```python
from build123d import *

# Parameters (mm, degrees)
BOSS_EXTRUDE2_DEPTH = 11.684
SKETCH3_R           = 12
CUT_EXTRUDE1_DEPTH  = 17.78
SKETCH5_R           = 4.7625
SKETCH5_R_2         = 3.96875
CUT_EXTRUDE3_DEPTH  = 24.368
SKETCH4_R           = 7.5
CUT_EXTRUDE2_DEPTH  = 24.368
CUT_EXTRUDE4_DEPTH  = 9.525
CUT_EXTRUDE5_DEPTH  = 9.525
SKETCH10_R          = 14
CUT_EXTRUDE6_DEPTH  = 1.905
CUT_EXTRUDE7_REACH  = 35.001
SKETCH12_W          = 38.1
SKETCH12_H          = 16.002
CUT_EXTRUDE8_REACH  = 32.013
SKETCH15_W          = 50.8
SKETCH15_H          = 17.5768
FILLET2_R           = 3.175
FILLET3_R           = 6.35
FILLET4_R           = 2.54
SKETCH16_R          = 17.272
CUT_EXTRUDE9_DEPTH  = 3.048


with BuildPart() as part:
    # Sketch2 → Boss-Extrude2 (new body, symmetric)
    with BuildSketch(Plane(origin=(0, 0, 0), x_dir=(1, 0, 0), z_dir=(0, 1, 0))):
        with BuildLine():
            Line((-42.844042296, 9.135566968), (24.187242381, 62.581479461))
            ThreePointArc((24.187242381, 62.581479461), (37.709893542, 62.836755255), (41.463262143, 49.842930403))
            Line((41.463262143, 49.842930403), (19.040802343, -7.451688072))
            ThreePointArc((19.040802343, -7.451688072), (9.340036317, -18.189104722), (-5.038725, -19.816434073))
            Line((-5.038725, -19.816434073), (-38.439271429, -11.323676613))
            ThreePointArc((-38.439271429, -11.323676613), (-46.982276413, -2.459157895), (-42.844042296, 9.135566968))
        make_face()
    extrude(amount=BOSS_EXTRUDE2_DEPTH, both=True)

    # Sketch3 → Cut-Extrude1 (cut)
    with BuildSketch(Plane.XZ.offset(11.684)):
        Circle(SKETCH3_R)
    extrude(amount=-CUT_EXTRUDE1_DEPTH, mode=Mode.SUBTRACT)

    # Sketch5 → Cut-Extrude3 (cut, through all)
    with BuildSketch(Plane(origin=(0, 11.684, 0), x_dir=(1, 0, 0), z_dir=(0, 1, 0))):
        with Locations((-35.56, 0)):
            Circle(SKETCH5_R)
        with Locations((31.115, 53.892760878)):
            Circle(SKETCH5_R_2)
    extrude(amount=-CUT_EXTRUDE3_DEPTH, mode=Mode.SUBTRACT)

    # Sketch4 → Cut-Extrude2 (cut, through all)
    with BuildSketch(Plane(origin=(0, 11.684, 0), x_dir=(1, 0, 0), z_dir=(0, 1, 0))):
        Circle(SKETCH4_R)
    extrude(amount=-CUT_EXTRUDE2_DEPTH, mode=Mode.SUBTRACT)

    # Sketch6 → Cut-Extrude4 (cut)
    with BuildSketch(Plane(origin=(0, 11.684, 0), x_dir=(1, 0, 0), z_dir=(0, 1, 0))):
        with BuildLine():
            Line((8.810645098, 41.106966719), (25.147527575, 31.674863223))
            ThreePointArc((25.147527575, 31.674863223), (27.965170287, 28.275776503), (27.885820228, 23.861413067))
            Line((27.885820228, 23.861413067), (23.481205903, 12.606595374))
            ThreePointArc((23.481205903, 12.606595374), (18.614262725, 8.65758593), (12.727975438, 10.810127095))
            ThreePointArc((12.727975438, 10.810127095), (1.647083767, 16.617680994), (-10.358254645, 13.098349791))
            ThreePointArc((-10.358254645, 13.098349791), (-20.167393041, 14.234267976), (-19.051094323, 24.045658467))
            Line((-19.051094323, 24.045658467), (1.676926459, 40.572687453))
            ThreePointArc((1.676926459, 40.572687453), (5.16139062, 41.939970615), (8.810645098, 41.106966719))
        make_face()
    extrude(amount=-CUT_EXTRUDE4_DEPTH, mode=Mode.SUBTRACT)

    # Sketch8 → Cut-Extrude5 (cut)
    with BuildSketch(Plane.XZ.offset(11.684)):
        with BuildLine():
            Line((25.147527575, -31.674863223), (8.810645098, -41.106966719))
            ThreePointArc((8.810645098, -41.106966719), (5.16139062, -41.939970615), (1.676926459, -40.572687453))
            Line((1.676926459, -40.572687453), (-13.415958874, -28.5387091))
            ThreePointArc((-13.415958874, -28.5387091), (-14.944664248, -20.378311947), (-7.092930176, -17.680295289))
            ThreePointArc((-7.092930176, -17.680295289), (4.120108003, -18.599118529), (13.896097136, -13.030770675))
            ThreePointArc((13.896097136, -13.030770675), (19.728139709, -11.138779489), (24.441422168, -15.060172058))
            Line((24.441422168, -15.060172058), (27.885820228, -23.861413067))
            ThreePointArc((27.885820228, -23.861413067), (27.965170287, -28.275776503), (25.147527575, -31.674863223))
        make_face()
    extrude(amount=-CUT_EXTRUDE5_DEPTH, mode=Mode.SUBTRACT)

    # Sketch10 → Cut-Extrude6 (cut)
    with BuildSketch(Plane(origin=(0, 11.684, 0), x_dir=(1, 0, 0), z_dir=(0, 1, 0))):
        Circle(SKETCH10_R)
    extrude(amount=-CUT_EXTRUDE6_DEPTH, mode=Mode.SUBTRACT)

    # Sketch12 → Cut-Extrude7 (cut, up to next)
    with BuildSketch(Plane(origin=(26.337597963, 0, -35.719049385), x_dir=(0.804858887, 0, 0.593466235), z_dir=(-0.593466235, 0, 0.804858887)), mode=Mode.PRIVATE) as cut_extrude7_sk1:
        with Locations((-6.94034966, 0)):
            Rectangle(SKETCH12_W, SKETCH12_H)
    cut_extrude7_tool1 = extrude(cut_extrude7_sk1.sketch, amount=-CUT_EXTRUDE7_REACH, mode=Mode.PRIVATE) & part.part
    add(cut_extrude7_tool1.solids().sort_by_distance((20.751596, 0, -39.837913))[0], mode=Mode.SUBTRACT)

    # Sketch15 → Cut-Extrude8 (cut, up to next)
    with BuildSketch(Plane(origin=(-20.01728519, 0, 4.309619478), x_dir=(0.210472261, 0, 0.97759983), z_dir=(-0.97759983, 0, 0.210472261)), mode=Mode.PRIVATE) as cut_extrude8_sk1:
        with Locations((-7.484393594, 0)):
            Rectangle(SKETCH15_W, SKETCH15_H)
    cut_extrude8_tool1 = extrude(cut_extrude8_sk1.sketch, amount=CUT_EXTRUDE8_REACH, mode=Mode.PRIVATE) & part.part
    add(cut_extrude8_tool1.solids().sort_by_distance((-21.592542, 0, -3.007122))[0], mode=Mode.SUBTRACT)

    # Fillet2
    fillet2_edges = [part.edges().sort_by_distance(p)[0] for p in [
        (19.728139709, -2.159, -11.138779489),
        (26.163621198, -2.159, -19.460792562),
        (27.965170287, -2.159, -28.275776503),
        (16.979086336, -2.159, -36.390914971),
        (5.16139062, -2.159, -41.939970615),
        (-5.869516208, -2.159, -34.555698277),
        (-14.944664248, -2.159, -20.378311947),
        (4.120108003, -2.159, -18.599118529),
    ]]
    fillet(fillet2_edges, radius=FILLET2_R)

    # Fillet3
    fillet3_edges = [part.edges().sort_by_distance(p)[0] for p in [
        (20.751595863, -8.001, -39.83791257),
        (20.751595863, 8.001, -39.83791257),
        (-21.59254243, -8.7884, -3.007122426),
        (-21.59254243, 8.7884, -3.007122426),
    ]]
    fillet(fillet3_edges, radius=FILLET3_R)

    # Fillet4
    fillet4_edges = [part.edges().sort_by_distance(p)[0] for p in [
        (-20.167393041, 2.159, -14.234267976),
        (-8.687083932, 2.159, -32.30917296),
        (5.16139062, 2.159, -41.939970615),
        (16.979086336, 2.159, -36.390914971),
        (27.965170287, 2.159, -28.275776503),
        (25.683513065, 2.159, -18.234004221),
        (18.614262725, 2.159, -8.65758593),
        (1.647083767, 2.159, -16.617680994),
    ]]
    fillet(fillet4_edges, radius=FILLET4_R)

    # Sketch16 → Cut-Extrude9 (cut)
    with BuildSketch(Plane.XZ.offset(11.684)):
        Circle(SKETCH16_R)
    extrude(amount=-CUT_EXTRUDE9_DEPTH, mode=Mode.SUBTRACT)


solid = part.part
```
The model under review builds one solid part; all positions refer to its coordinate system, in mm. A direction names the side the tool comes from. Give positions to 0.01 mm unless a question says otherwise; leave off trailing zeros. Write each loop counter-clockwise with the first axis right and the second up, starting at its lowest first coordinate (ties: lowest second). Pieces come first, ordered by that corner, then holes. Notation, with made-up numbers: M 76,-39 L 135,-39 A22 cw 135,-16 Z; hole C 26.25,66 d4. An arc over 180 degrees is marked long. Write item = value, one per line. Start each with the question number.
Q1. For line 1 (Y direction, x = 35, z = -55.5); line 2 (X direction, y = 10.4, z = 0); line 3 (Z direction, x = 0, y = -10.05), list the stretches that pass through material, from the lowest coordinate up.
Q2. Mouldability with a two-part tool opening along Y and no side actions: class faces 1 (the face through (37.54, 9.87, -62.96)), 2 (the face through (-21.65, 0.03, -3.28)), 3 (the face through (24.978, 2.923, -18.419)) as released by +Y, released by -Y, zero draft, split by the parting line, or undercut.
Q3. Clearance check with flat-ended pins moving along their axes: pin 1 (1.5 mm diameter, centred on x = -6.5, y = 7, fed in from +Z); pin 2 (14 mm diameter, centred on x = -6.5, z = 5, fed in from +Y); pin 3 (8 mm diameter, centred on y = 4.5, z = -29, fed in from -X); pin 4 (5 mm diameter, centred on x = -7.5, z = -1, fed in from +Y). State where each tip first meets the part, or that it passes through.
Q4. We need section C-C (z = -2.5). Give the number of separate pieces and of enclosed holes in the cut face, plus the area to 3 significant figures.
Q5. We need section B-B (z = -56.5). State the section outline as (x, y) points, plus the area to 3 significant figures.
Q6. We need section A-A (x = -35.56). State the section outline as (y, z) points.
Q7. Machinability: for faces 4 (the face through (-39, -8.788, 4)), 5 (the face through (22.07, 6.19, -41.24)), 6 (the face through (-20.071, 8.24, -14.115)), which of the approach directions +Z, -Z, +X, -X, +Y, -Y give a long, thin tool a straight path to every point of the face, cutting with its end or side? Answer none if there is none.
Result set:
q1.line_1 = -11.68 to -8, 8 to 11.68
q1.line_2 = -47.24 to -40.32, -30.8 to -14, 14 to 21.96
q1.line_3 = -43.3 to -39.24, -19.05 to -17.27, 17.27 to 20.45
q2.face_1 = zero draft
q2.face_2 = undercut
q2.face_3 = released by +Y
q3.pin_1 = 19.64
q3.pin_2 = 11.68
q3.pin_3 = -22.95
q3.pin_4 = 9.78
q4.separate_pieces = 4
q4.enclosed_holes = 0
q4.area = 602 mm2
q5.outline = M 16.56,-11.68 L 28.12,-11.68 L 28.12,-8 L 16.56,-8 Z; M 16.56,8 L 28.12,8 L 28.12,11.68 L 16.56,11.68 Z; M 34.11,-11.68 L 41.92,-11.68 L 41.92,-8 L 34.11,-8 Z; M 34.11,8 L 41.92,8 L 41.92,11.68 L 34.11,11.68 Z
q5.area = 143 mm2
q6.outline = M -11.68,-14.94 L -8.79,-14.94 L -8.79,-4.76 L -11.68,-4.76 Z; M -11.68,4.76 L -8.79,4.76 L -8.79,12.06 L -11.68,12.06 Z; M 8.79,-14.94 L 11.68,-14.94 L 11.68,-4.76 L 8.79,-4.76 Z; M 8.79,4.76 L 11.68,4.76 L 11.68,12.06 L 8.79,12.06 Z
q7.face_4 = +Z, -X
q7.face_5 = -Z, +X
q7.face_6 = +Y
